The listing builds one solid part. Answer for the finished solid, in the listing's coordinates (mm). Give positions to 0.01 mm unless a question says otherwise; leave off trailing zeros. Order: outer loops, then holes, each group sorted by start corner. A loop starts at its lowest first (then second) coordinate and runs counter-clockwise, first axis right, second up. Notation, with made-up numbers: (12.25, 27.25) - (65.25, 27.25) arc R6 cw to (65.25, 38.25) - close; hole circle Ø6 at (-10, -40). An arc over 180 degrees is marked (long way). Use a Markdown table: item, result. Add a question column.
1) A flat-ended cylindrical pin translates along its axis: pin 1 (5 mm diameter, centred on x = 6, y = -3.5, fed in from -Z). Find the tip coordinate at first contact, or state that the pin passes through.
2) Find section B-B, the plane y = -8.25. Determine the outline of the cut face in (x, z).
3) Find section A-A, the plane z = 3.5. Determine the outline of the cut face in (x, y), plus the area to 3 significant figures.
4) Straight lines are drawn through the part: line 1 (Z direction, x = 4.5, y = -7.25); line 2 (X direction, y = -5, z = 5.25); line 3 (Y direction, x = 8.75, z = 1.5). For each, find the intervals that lie inside material, in ascending order.
Autodesk Inventor part; units mm, degrees
ref_plane "YZ Plane" through (0, 0, 0) normal (1, 0, 0) x (0, 1, 0)
ref_plane "XZ Plane" through (0, 0, 0) normal (0, 1, 0) x (-1, 0, 0)
ref_plane "XY Plane" through (0, 0, 0) normal (0, 0, 1) x (1, 0, 0)
sketch "Sketch1" plane through (0, 0, 0) normal (0, 0, 1) x (1, 0, 0)
  line L0 (0, 0) -> (11.9888, 0)
  line L1 (11.9888, 0) -> (11.9888, -10.0076)
  line L2 (11.9888, -10.0076) -> (0, -10.0076)
  line L3 (0, -10.0076) -> (0, 0)
  dimension "d0" = 10.0076
  dimension "d1" = 11.9888
extrude "Extrusion1" add sketch "Sketch1" along normal blind 10.0076
shell "Shell1" thickness 1.27 removed faces 1 at (3.9963, -6.6717, 10.0076)
sketch "Sketch2" plane through (0, 0, 10.0076) normal (0, 0, 1) x (1, 0, 0)
  line L0 (1.27, -1.27) -> (10.7188, -1.27)
  line L1 (10.7188, -1.27) -> (10.7188, -8.7376)
  line L2 (10.7188, -8.7376) -> (1.27, -8.7376)
  line L3 (1.27, -8.7376) -> (1.27, -1.27)
extrude "Extrusion2" add sketch "Sketch2" against normal blind 3.81
properties part number "Gearmotor_Gear" material "Brass, Soft Yellow"
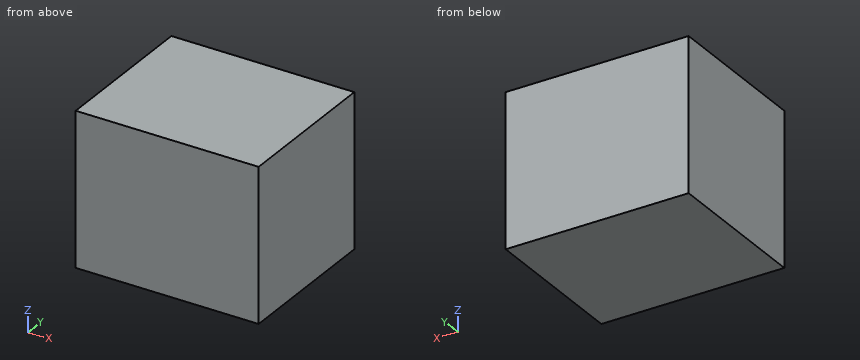
The answers:
| question | item | result |
|---|---|---|
| 1 | pin 1 | z = 0 |
| 2 | outline | (0, 0) - (11.99, 0) - (11.99, 10.01) - (0, 10.01) - close; hole (1.27, 1.27) - (10.72, 1.27) - (10.72, 6.2) - (1.27, 6.2) - close |
| 3 | outline | (0, -10.01) - (11.99, -10.01) - (11.99, 0) - (0, 0) - close; hole (1.27, -8.74) - (10.72, -8.74) - (10.72, -1.27) - (1.27, -1.27) - close |
| 3 | area | 49.4 mm2 |
| 4 | line 1 | 0 to 1.27, 6.2 to 10.01 |
| 4 | line 2 | 0 to 1.27, 10.72 to 11.99 |
| 4 | line 3 | -10.01 to -8.74, -1.27 to 0 |
